Could you check a few things on this model? Use its own coordinates, in mm. A direction names the side the tool comes from. Give positions to 0.01 mm unless a question says otherwise; leave off trailing zeros. Order: outer loops, then holes, each group sorted by start corner. A loop starts at its lowest first (then second) coordinate and runs counter-clockwise, first axis right, second up. Notation, with made-up numbers: M -37,34.5 L -1,34.5 A21 ccw -1,41.5 Z; hole C 34,-5.75 d1. An arc over 180 degrees is marked long. Return JSON: item names as keys, results as strings. Group by question number.
```python
from build123d import *

# Parameters (mm, degrees)
SKETCH_2_R          = 5
CUT_EXTRUDE_1_DEPTH = 74.484692283


with BuildPart() as part:
    # Эскиз1 → Повернуть1 (revolve)
    with BuildSketch(Plane(origin=(0, 0, 0), x_dir=(0, 0, -1), z_dir=(1, 0, 0)), mode=Mode.PRIVATE) as revolve_1_sk:
        with BuildLine():
            Line((6, 50), (10, 50))
            Line((10, 50), (10, 40))
            Line((10, 40), (5, 35))
            Line((5, 35), (5, 15))
            Line((5, 15), (10, 15))
            Line((10, 15), (10, 0))
            Line((10, 0), (-10, 0))
            Line((-10, 0), (-10, 15))
            Line((-10, 15), (-5, 15))
            Line((-5, 15), (-5, 35))
            Line((-5, 35), (-10, 40))
            Line((-10, 40), (-10, 50))
            Line((-10, 50), (-6, 50))
            ThreePointArc((-6, 50), (0, 44), (6, 50))
        make_face()
    revolve(revolve_1_sk.sketch.rotate(Axis((0, 0, 10), (0, 0, -1)), 180), axis=Axis((0, 0, 10), (0, 0, -1)))

    # Эскиз2 → Вырез-Вытянуть1 (cut, through all)
    with BuildSketch(Plane.XY.offset(10)):
        Circle(SKETCH_2_R)
    extrude(amount=-CUT_EXTRUDE_1_DEPTH, mode=Mode.SUBTRACT)


solid = part.part
```
1. Imagine slicing it at B-B, the plane z = 7.5. Please give me the cut outline in (x, y), plus the area to 3 significant figures.
2. I need wall thicknesses on L1, parallel to Z at x = -5, y = 23.5; L2, parallel to X at y = -30.5, z = 8.25; L3, parallel to Y at x = -16.5, z = 7.5. Which ranges of each line are inside material? Lowest first, please. Write a range as from..to.
3. Which directions (+Z, -Z, +X, -X, +Y, -Y) give clear straight access to the entire face, cutting with the end or side of a thin tool? Please do faces 1 (the flat face through (-4, -4, 10)), 2 (the flat face through (7, -15, -5)), 3 (the flat face through (7, 15, 5)).
4. For pin 1 (12 mm diameter, centred on x = -19.5, y = -2.5, fed in from -Z); pin 2 (8 mm diameter, centred on x = -5.5, z = -0.5, fed in from +Y); pin 3 (4 mm diameter, centred on y = 13.5, z = 7, fed in from +X); pin 4 (4 mm diameter, centred on x = 23, y = 12.5, fed in from -Z), each with a flat end and sliding along its axis, tell me the tip position at first contact or that it passes through.
5. Imagine slicing it at A-A, the plane x = 0. Please give me the cut outline in (y, z), plus the area to 3 significant figures.
6. Imagine slicing it at C-C, the plane z = 1.5. Please give me the cut outline in (x, y).
Values:
{
 "1": {"outline": "C 0,0 d100; C 0,0 d30; hole C 0,0 d75; hole C 0,0 d10", "area": "4,060 mm²"},
 "2": {"L1": "z = -5..5", "L2": "x = -39.62..-23.08, 23.08..39.62", "L3": "y = -47.2..-33.67, 33.67..47.2"},
 "3": {"face 1": "+Z, +X, -X, +Y, -Y", "face 2": "-Z", "face 3": "+Z"},
 "4": {"pin 1": "stops at z = -10", "pin 2": "stops at y = 45.73", "pin 3": "stops at x = 48.66", "pin 4": "stops at z = -5"},
 "5": {"outline": "M -50,-10 L -40,-10 L -35,-5 L -15,-5 L -15,-10 L -5,-10 L -5,10 L -15,10 L -15,5 L -35,5 L -40,10 L -50,10 L -50,6 A6 cw -50,-6 Z; M 5,-10 L 15,-10 L 15,-5 L 35,-5 L 40,-10 L 50,-10 L 50,-6 A6 cw 50,6 L 50,10 L 40,10 L 35,5 L 15,5 L 15,10 L 5,10 Z", "area": "1,240 mm²"},
 "6": {"outline": "C 0,0 d88.38; hole C 0,0 d10"}
}
